Drawing for the job (mm, zero at the part's lowest x, y, z). Coordinates: 2 decimals unless noted, no trailing zeros. Write each loop counter-clockwise with the first axis right and the second up, starting at its lowest first coordinate (ties: lowest second). Pieces come first, ordered by that corner, then holes. Notation, with made-up numbers: (19, -9) -> (71, -9) arc R16 ccw to (71, 18) -> close; hole circle Ø3 at (61.5, -3.5). An arc over 180 degrees is marked (long way). Answer as CSV lines item,"result". Start each with the question number.
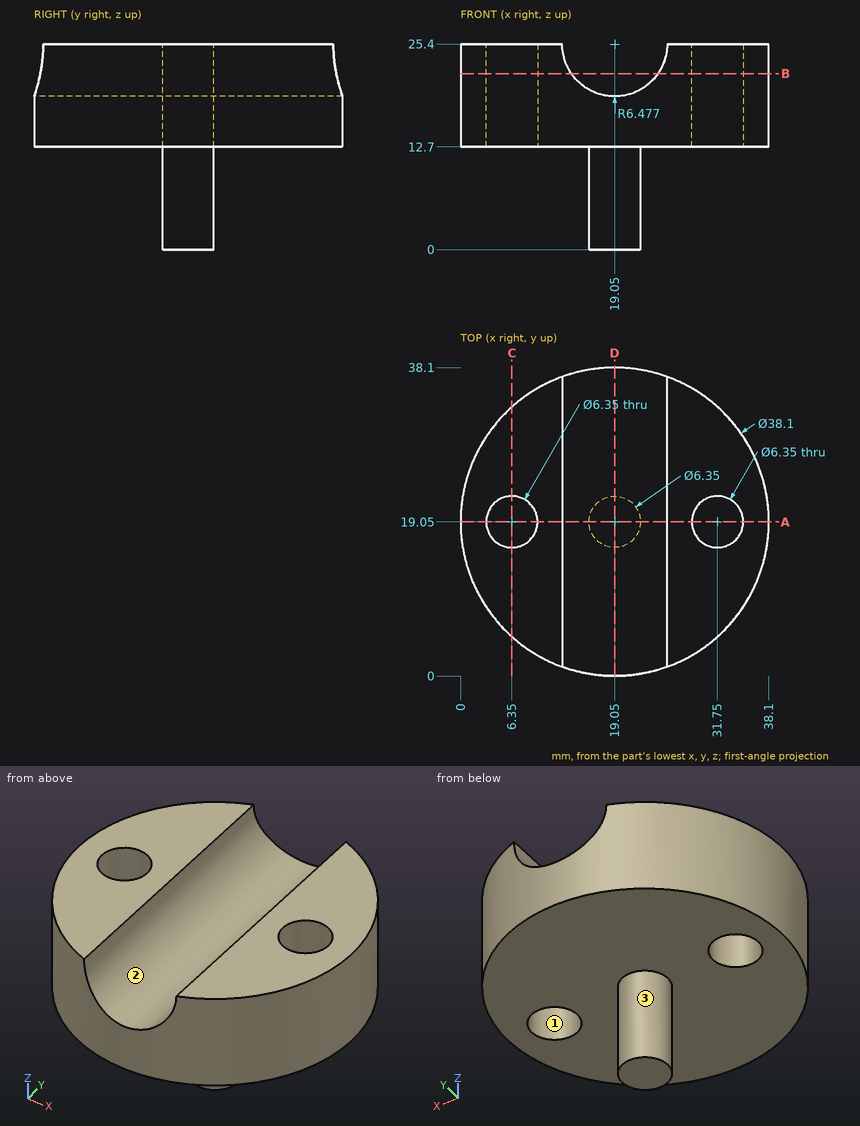
1. Wall check: line 1 (Z direction, x = 27.5, y = 20.5); line 2 (X direction, y = 14.5, z = 20.25); line 3 (Y direction, x = 31.75, z = 15.5) (3 decimals). Give the ranges that are in metal, low to high.
2. Flat gauge pins, fed straight in: P1, Ø6, axis at y = 32, z = 14, coming from the +X side (3 decimals); P2, Ø5, axis at y = 26, z = 21, coming from the -X side; P3, Ø7.5, axis at x = 6.35, y = 19.05, coming from the +Z side; P4, Ø2, axis at x = 14, z = 18, coming from the -Y side. Where does each tip first touch, or does it go through?
3. Cut at B-B (z = 21.75). Give the cut face in (x, y) (3 decimals), then the cut area to 3 significant figures.
4. Mould opens along Y. For the marked faces 1, 2 and 3 say: pulls with the +Y half, pulls with the -Y half, needs draft (parallel to the pull), parting line crosses it, or undercut.
5. Cut at D-D (x = 19.05). Give the cut face in (y, z) (3 decimals).
6. Cut at C-C (x = 6.35). Give the cut face in (y, z) (3 decimals), then the cut area to 3 significant figures.
7. Cut at A-A (y = 19.05). Give the cut face in (x, z) (3 decimals).
Geometry check:
1,line 1,"12.7 to 25.4"
1,line 2,"0.55 to 15.12, 22.98 to 37.55"
1,line 3,"4.851 to 15.875, 22.225 to 33.249"
2,P1,"x = 35.295"
2,P2,"x = 0.53"
2,P3,"z = 25.4"
2,P4,"y = 0.44"
3,outline,"(13.699, 0.767) -> (13.699, 37.333) arc R19.05 ccw to start; (24.401, 0.767) arc R19.05 ccw to (24.401, 37.333) -> close; hole circle Ø6.35 at (6.35, 19.05); hole circle Ø6.35 at (31.75, 19.05)"
3,area,"674 mm²"
4,face 1,"undercut"
4,face 2,"needs draft"
4,face 3,"parting line crosses it"
5,outline,"(0, 12.7) -> (15.875, 12.7) -> (15.875, 0) -> (22.225, 0) -> (22.225, 12.7) -> (38.1, 12.7) -> (38.1, 18.923) -> (0, 18.923) -> close"
6,outline,"(4.851, 12.7) -> (15.875, 12.7) -> (15.875, 25.4) -> (4.851, 25.4) -> close; (22.225, 12.7) -> (33.249, 12.7) -> (33.249, 25.4) -> (22.225, 25.4) -> close"
6,area,"280 mm²"
7,outline,"(0, 12.7) -> (3.175, 12.7) -> (3.175, 25.4) -> (0, 25.4) -> close; (9.525, 12.7) -> (15.875, 12.7) -> (15.875, 0) -> (22.225, 0) -> (22.225, 12.7) -> (28.575, 12.7) -> (28.575, 25.4) -> (25.527, 25.4) arc R6.477 cw to (12.573, 25.4) -> (9.525, 25.4) -> close; (34.925, 12.7) -> (38.1, 12.7) -> (38.1, 25.4) -> (34.925, 25.4) -> close"
